Model file for the job. Use its own axes, mm. Round coordinates to 2 decimals unless told otherwise and drop trailing zeros. Order: outer loops, then holes, each group sorted by start corner. A loop starts at its lowest first (then second) coordinate and runs counter-clockwise, first axis right, second up. Notation, with made-up numbers: (34.25, -22) - (43.25, -22) arc R14 cw to (43.25, -9) - close; hole circle Ø1 at (64.5, -7). An arc over 180 degrees is marked (long way). Answer as CSV lines item,"result". Start each with the question number.
1. Wall check: line 1 along Z through (x, y) = (-38, -1.5); line 2 along Z through (x, y) = (-34.5, -2.6); line 3 along X through (y, z) = (-2.65, 0). Give the ranges that are in metal, low to high. Write a range as [from, to].
2. Band-saw the part on C-C on x = -1.5. List the corners of the cut face in (y, z), then the cut area to 3 significant figures.
3. Band-saw the part on B-B on z = 22. List the corners of the cut face in (x, y).
4. Band-saw the part on A-A on y = -2. State how many separate pieces and enclosed holes the cut face has, then the cut area to 3 significant figures.
5. Pin check, flat tips, straight feed: pin 1 Ø1 at (x, y) = (-35.5, -1) entering from -Z; pin 2 Ø0.9 at (y, z) = (-2, 17.5) entering from +X. Stop position of each tip, or through.
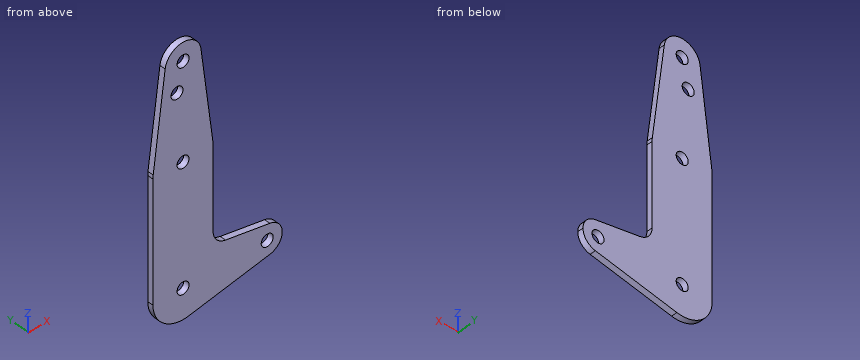
```python
from build123d import *

# Parameters (mm, degrees)
F0_R     = 3.175
F1_DEPTH = 3.048


with BuildPart() as f1:
    # F0 (on Front) → F1 (new body)
    with BuildSketch(Plane.XZ):
        with BuildLine():
            ThreePointArc((-27.823383, 88.464874), (-27.767371, 87.870732), (-27.748676, 87.274249))
            ThreePointArc((-27.748676, 87.274249), (-37.870159, 77.767944), (-46.723969, 88.464874))
            Line((-46.723969, 88.464874), (-53.024164, 38.458624))
            ThreePointArc((-53.024164, 38.458624), (-37.273676, 52.349249), (-21.523187, 38.458624))
            Line((-21.523187, 38.458624), (-27.823383, 88.464874))
        make_face()
        with Locations((-40.448676, 72.999449)):
            Circle(F0_R, mode=Mode.SUBTRACT)
        with BuildLine():
            ThreePointArc((-46.723969, 88.464874), (-37.870159, 77.767944), (-27.748676, 87.274249))
            ThreePointArc((-27.748676, 87.274249), (-27.767371, 87.870732), (-27.823383, 88.464874))
            ThreePointArc((-27.823383, 88.464874), (-37.273676, 96.799249), (-46.723969, 88.464874))
        make_face()
        with Locations((-37.273676, 87.274249)):
            Circle(F0_R, mode=Mode.SUBTRACT)
        with BuildLine():
            ThreePointArc((-21.398676, 36.474249), (-21.429834, 37.468387), (-21.523187, 38.458624))
            ThreePointArc((-21.523187, 38.458624), (-37.273676, 52.349249), (-53.024164, 38.458624))
            ThreePointArc((-53.024164, 38.458624), (-53.117517, 37.468387), (-53.148676, 36.474249))
            ThreePointArc((-53.148676, 36.474249), (-37.273676, 20.599249), (-21.398676, 36.474249))
        make_face()
        with Locations((-37.273676, 36.474249)):
            Circle(F0_R, mode=Mode.SUBTRACT)
        with BuildLine():
            Line((-21.398676, -7.135352), (-21.398676, 36.474249))
            ThreePointArc((-21.398676, 36.474249), (-37.273676, 20.599249), (-53.148676, 36.474249))
            Line((-53.148676, 36.474249), (-53.148676, -27.025751))
            ThreePointArc((-53.148676, -27.025751), (-37.273676, -11.150751), (-21.398676, -27.025751))
            ThreePointArc((-21.398676, -27.025751), (-25.08724, -37.199562), (-34.438854, -42.645592))
            Line((-34.438854, -42.645592), (8.593735, -34.835671))
            ThreePointArc((8.593735, -34.835671), (-0.761176, -27.025751), (8.593735, -19.215831))
            Line((8.593735, -19.215831), (-14.868154, -14.957768))
            ThreePointArc((-14.868154, -14.957768), (-19.551442, -12.230396), (-21.398676, -7.135352))
        make_face()
        with BuildLine():
            ThreePointArc((-21.398676, -27.025751), (-37.273676, -11.150751), (-53.148676, -27.025751))
            ThreePointArc((-53.148676, -27.025751), (-47.447486, -39.212187), (-34.438854, -42.645592))
            ThreePointArc((-34.438854, -42.645592), (-25.08724, -37.199562), (-21.398676, -27.025751))
        make_face()
        with Locations((-37.273676, -27.025751)):
            Circle(F0_R, mode=Mode.SUBTRACT)
        with BuildLine():
            ThreePointArc((15.113824, -27.025751), (13.269542, -21.938846), (8.593735, -19.215831))
            ThreePointArc((8.593735, -19.215831), (-0.761176, -27.025751), (8.593735, -34.835671))
            ThreePointArc((8.593735, -34.835671), (13.269542, -32.112656), (15.113824, -27.025751))
        make_face()
        with Locations((7.176324, -27.025751)):
            Circle(F0_R, mode=Mode.SUBTRACT)
    extrude(amount=F1_DEPTH)


solid = f1.part
```
Reply:
1,line 1,"z = [-42.88, -30.12], [-23.93, 33.38], [39.57, 70.98], [75.02, 84.18], [90.37, 96.77]"
1,line 2,"z = [-42.66, -28.57], [-25.48, 34.93], [38.02, 85.73], [88.82, 96.39]"
1,line 3,"x = [-53.15, -21.4]"
2,outline,"(-3.05, -36.67) - (0, -36.67) - (0, -17.38) - (-3.05, -17.38) - close"
2,area,"58.8 mm2"
3,outline,"(-53.15, -3.05) - (-21.4, -3.05) - (-21.4, 0) - (-53.15, 0) - close"
4,separate pieces,"1"
4,enclosed holes,"5"
4,area,"4,450 mm2"
5,pin 1,"stops at z = -42.85"
5,pin 2,"stops at x = -21.4"
